Verification items for the finished model (mm, model axes). A direction names the side the tool comes from. Give positions to 0.01 mm unless a question says otherwise; leave off trailing zeros. Order: outer loops, then holes, each group sorted by start corner. A loop starts at its lowest first (then second) coordinate and runs counter-clockwise, first axis right, second up. Notation, with made-up numbers: (57.25, -16) -> (105.25, -16) arc R19 ccw to (105.25, -10) -> close; hole circle Ø9 at (2.5, 26). An arc over 180 degrees is marked (long way). Write each question's results on one line, items separated by ' | '. Start each with the question number.
1. Cross-section at D-D, the plane y = 43. Enter the section's corners in (x, z).
2. Material ranges on L1, parallel to Z at x = 38, y = 25; L2, parallel to Z at x = 48.5, y = 7; L3, parallel to X at y = 26, z = 13.75, recorded low to high. Write a range as from..to.
3. Cross-section at B-B, the plane y = 35.5. Enter the section's corners in (x, z), then the cut area to 3 significant figures.
4. Set-up check for faces 1 (the face through (1.752, 56.287, 13.493)), 2 (the face through (71.287, 56.248, 13.493)), 3 (the face through (66.08, 4.01, 14.81)), 4 (the face through (36, 58, 6)), 5 (the face through (71.248, 8.713, 13.493)): record each of +Z, -Z, +X, -X, +Y, -Y from which the full face is reachable in a straight line by a thin tool's end or side.
5. Cross-section at C-C, the plane x = 38. Enter the section's corners in (y, z).
6. Mould release check, pull along Y, two halves, no side actions. Record for faces 6 (the face through (37, 45, 1)), 7 (the face through (72, 56.95, 6.59)), 8 (the face through (36, 29, 0)), 9 (the face through (1.713, 8.752, 13.493)): +Y half, -Y half, draft (parallel to the pull), parting line (faces both ways), or undercut.
7. Depth check by flat-ended pin: pin 1 Ø10 at (x, y) = (14.5, 35.5) entering from +Z; pin 2 Ø0.5 at (y, z) = (28, 13.5) entering from +X; pin 3 Ø0.8 at (x, z) = (69, 13.5) entering from -Y. Enter the tip coordinate at first touch or a pass-through.
8. Cross-section at A-A, the plane x = 64. Enter the section's corners in (y, z).
from build123d import *

# Parameters (mm, degrees)
SKETCH1_W           = 73
SKETCH1_H           = 58
BOSS_EXTRUDE1_DEPTH = 13
FILLET1_R           = 3.5
BOSS_EXTRUDE2_DEPTH = 1
SKETCH3_R           = 4.5
BOSS_EXTRUDE3_DEPTH = 3
SKETCH6_W           = 53
SKETCH6_H           = 6
CUT_EXTRUDE2_DEPTH  = 1


with BuildPart() as part:
    # Sketch1 → Boss-Extrude1 (new body)
    with BuildSketch(Plane.XY):
        with Locations((36.5, 29)):
            Rectangle(SKETCH1_W, SKETCH1_H)
    extrude(amount=BOSS_EXTRUDE1_DEPTH)

    # Fillet1
    fillet1_edges = [part.edges().sort_by_distance(p)[0] for p in [
        (0, 58, 6.5),
        (73, 58, 6.5),
        (73, 0, 6.5),
        (0, 0, 6.5),
    ]]
    fillet(fillet1_edges, radius=FILLET1_R)

    # Sketch2 → Boss-Extrude2 (add)
    with BuildSketch(Plane.XY.offset(13)):
        with BuildLine():
            Line((3.5, 8), (69.5, 8))
            ThreePointArc((69.5, 8), (71.267766953, 8.732233047), (72, 10.5))
            Line((72, 10.5), (72, 54.5))
            ThreePointArc((72, 54.5), (71.267766953, 56.267766953), (69.5, 57))
            Line((69.5, 57), (3.5, 57))
            ThreePointArc((3.5, 57), (1.732233047, 56.267766953), (1, 54.5))
            Line((1, 54.5), (1, 10.5))
            ThreePointArc((1, 10.5), (1.732233047, 8.732233047), (3.5, 8))
        make_face()
    extrude(amount=BOSS_EXTRUDE2_DEPTH)

    # Sketch3 → Boss-Extrude3 (add)
    with BuildSketch(Plane.XY.offset(13)):
        with Locations((64, 8)):
            Circle(SKETCH3_R)
    extrude(amount=BOSS_EXTRUDE3_DEPTH)

    # Sketch6 → Cut-Extrude2 (cut)
    with BuildSketch(Plane(origin=(0, 0, 0), x_dir=(-1, 0, 0), z_dir=(0, 0, -1))):
        with Locations((-36.5, 45)):
            Rectangle(SKETCH6_W, SKETCH6_H)
    extrude(amount=-CUT_EXTRUDE2_DEPTH, mode=Mode.SUBTRACT)


solid = part.part
Results below:
1) outline: (0, 0) -> (10, 0) -> (10, 1) -> (63, 1) -> (63, 0) -> (73, 0) -> (73, 13) -> (72, 13) -> (72, 14) -> (1, 14) -> (1, 13) -> (0, 13) -> close
2) L1: z = 0..14 | L2: z = 0..13 | L3: x = 1..72
3) outline: (0, 0) -> (73, 0) -> (73, 13) -> (72, 13) -> (72, 14) -> (1, 14) -> (1, 13) -> (0, 13) -> close | area: 1,020 mm²
4) face 1: +Z, -X, +Y | face 2: +Z, +X, +Y | face 3: +Z | face 4: +Z, -Z, +X, -X, +Y | face 5: +Z, +X, -Y
5) outline: (0, 0) -> (42, 0) -> (42, 1) -> (48, 1) -> (48, 0) -> (58, 0) -> (58, 13) -> (57, 13) -> (57, 14) -> (8, 14) -> (8, 13) -> (0, 13) -> close
6) face 6: undercut | face 7: +Y half | face 8: draft | face 9: -Y half
7) pin 1: stops at z = 14 | pin 2: stops at x = 72 | pin 3: stops at y = 8
8) outline: (0, 0) -> (58, 0) -> (58, 13) -> (57, 13) -> (57, 14) -> (12.5, 14) -> (12.5, 16) -> (3.5, 16) -> (3.5, 13) -> (0, 13) -> close
